Geometry: final body of the model. Coordinates: model frame, mm. Give positions to 0.01 mm unless a question says otherwise; leave off trailing zeros. Write each loop counter-clockwise with the first axis right and the second up, starting at its lowest first coordinate (ties: lowest second). Pieces come first, ordered by that corner, then holes. Notation, with made-up numbers: (13, 22.5) -> (65, 22.5) arc R32 cw to (65, 51.5) -> close; hole circle Ø1 at (7.5, 19.5). An arc over 180 degrees is marked (long way). Answer as a JSON object with one key per item and string values.
from build123d import *

# Parameters (mm, degrees)
SKETCH1_R           = 2
SKETCH1_R_2         = 2.5
BOSS_EXTRUDE1_DEPTH = 3
FILLET2_R           = 3
FILLET3_R           = 3
SKETCH2_W           = 22
SKETCH2_H           = 12
CUT_EXTRUDE1_DEPTH  = 10


with BuildPart() as part:
    # Sketch1 → Boss-Extrude1 (new body)
    with BuildSketch(Plane(origin=(0, 0, 0), x_dir=(1, 0, 0), z_dir=(0, 1, 0))):
        with BuildLine():
            ThreePointArc((1.186783721, 19.964757559), (-20, 0), (1.186783721, -19.964757559))
            Line((1.186783721, -19.964757559), (168.819660113, -10))
            ThreePointArc((168.819660113, -10), (195, 0), (168.819660113, 10))
            Line((168.819660113, 10), (1.186783721, 19.964757559))
        make_face()
        with Locations(Location((60, 0, 0), (0, 0, 270))):
            Circle(SKETCH1_R, mode=Mode.SUBTRACT)
        with Locations(Location((0, 0, 0), (0, 0, 270))):
            Circle(SKETCH1_R_2, mode=Mode.SUBTRACT)
        with Locations(Location((120, 0, 0), (0, 0, 270))):
            Circle(SKETCH1_R, mode=Mode.SUBTRACT)
    extrude(amount=BOSS_EXTRUDE1_DEPTH)

    # Fillet2
    fillet2_edges = [part.edges().sort_by_distance(p)[0] for p in [
        (168.819660113, 1.5, -10),
    ]]
    fillet(fillet2_edges, radius=FILLET2_R)

    # Fillet3
    fillet3_edges = [part.edges().sort_by_distance(p)[0] for p in [
        (168.819660113, 1.5, 10),
    ]]
    fillet(fillet3_edges, radius=FILLET3_R)

    # Sketch2 → Cut-Extrude1 (cut)
    with BuildSketch(Plane(origin=(0, 3, 0), x_dir=(1, 0, 0), z_dir=(0, 1, 0))):
        with Locations((173, 0)):
            Rectangle(SKETCH2_W, SKETCH2_H)
    extrude(amount=-CUT_EXTRUDE1_DEPTH, mode=Mode.SUBTRACT)


solid = part.part
Q1. Material intervals for L1, parallel to Z at x = 153, y = 0.5; L2, parallel to Z at x = 17, y = 2, sorted ascending. Write a range as from..to.
Values:
{"L1": "-10.94..10.94", "L2": "-19.02..19.02"}
Q2. Cut plane C-C (x = 60). Return the cut outline in (y, z), and give its area (3 significant figures).
Values:
{"outline": "(0, -16.47) -> (3, -16.47) -> (3, -2) -> (0, -2) -> close; (0, 2) -> (3, 2) -> (3, 16.47) -> (0, 16.47) -> close", "area": "86.8 mm²"}
Q3. Cut plane D-D (x = 155). Return the cut outline in (y, z).
Values:
{"outline": "(0, -10.82) -> (3, -10.82) -> (3, 10.82) -> (0, 10.82) -> close"}
Q4. First-contact query: P1, Ø0.9, axis at y = 1.5, z = -1.5, coming from the -X side; P2, Ø1, axis at y = 1, z = 10.5, coming from the -X side; P3, Ø1.5, axis at x = 177, y = 1.5, coming from the +Z side. Flat tips, straight axial feed; report the tip coordinate or a pass-through.
Values:
{"P1": "x = -19.97", "P2": "x = -17.32", "P3": "z = 14.83"}
Q5. Cut plane A-A (x = 180). Return the cut outline in (y, z), and give its area (3 significant figures).
Values:
{"outline": "(0, -15) -> (3, -15) -> (3, -6) -> (0, -6) -> close; (0, 6) -> (3, 6) -> (3, 15) -> (0, 15) -> close", "area": "54.0 mm²"}
Q6. Mould query, pull axis Z, two halves, no side actions, for faces 1 (the flat face through (83.16, 1.48, 15.09)), 2 (the cylindrical face through (-2.44, 1.48, -0.54)), 3 (the flat face through (85.483, 1.479, -14.954)), 4 (the cylindrical face through (62, 1, 0)). Classes: pulls with the +Z half, pulls with the -Z half, needs draft (parallel to the pull), parting line crosses it, or undercut.
Values:
{"face 1": "pulls with the +Z half", "face 2": "undercut", "face 3": "pulls with the -Z half", "face 4": "undercut"}
Q7. Cut plane B-B (y = 0.85). Return the cut outline in (x, z).
Values:
{"outline": "(1.19, -19.96) -> (167.45, -10.08) arc R3 cw to (169.69, -10.9) arc R15 ccw (long way) to (169.69, 10.9) arc R3 cw to (167.45, 10.08) -> (1.19, 19.96) arc R20 ccw (long way) to start; hole circle Ø5 at (0, 0); hole circle Ø4 at (60, 0); hole circle Ø4 at (120, 0); hole (162, -6) -> (184, -6) -> (184, 6) -> (162, 6) -> close"}
